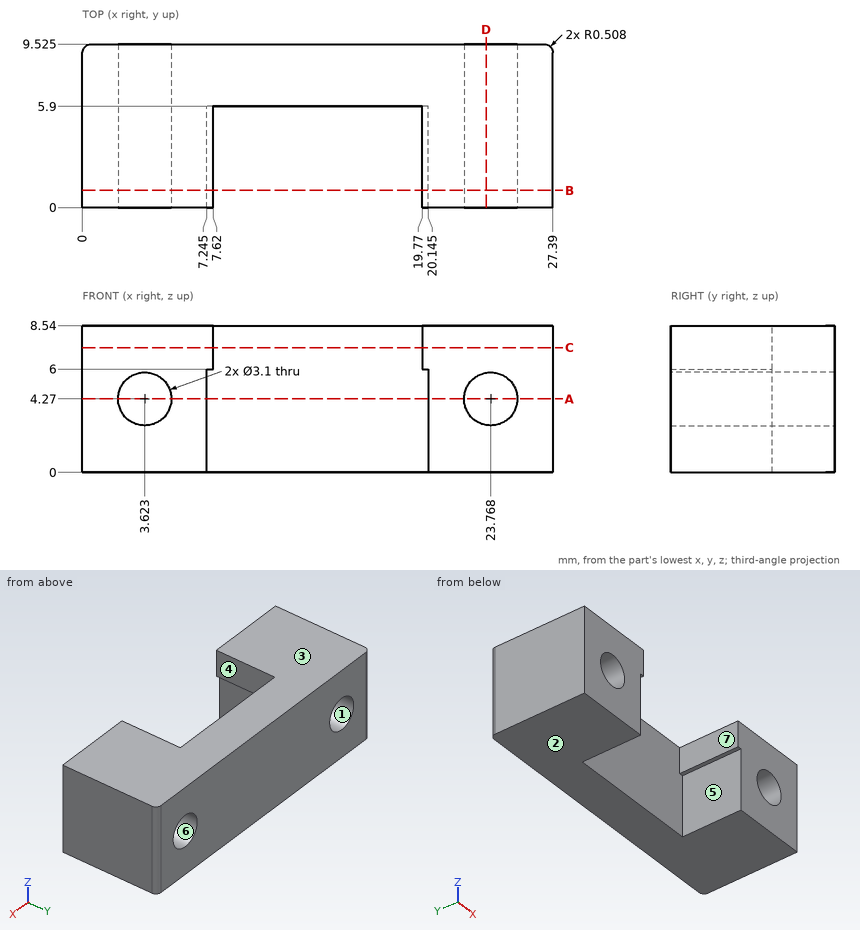
For this review, use the dimensioned drawing (mm, ordinates from the lowest corner) and the shaded views. A direction names the side the tool comes from. Coordinates: 2 decimals unless noted, no trailing zeros. Loops run counter-clockwise (first coordinate to the right, second up) from the corner with the lowest first, then second, coordinate; pieces in that order, holes last. Notation, with made-up numbers: (-31, 79.5) -> (-20, 79.5) arc R20 cw to (-20, 95.5) -> close; hole circle Ø7 at (62, 73.25). An arc over 180 degrees is marked (long way). Use a Markdown table: item, result. Add a question column.
Item 1: The part is to be moulded in two halves that separate along Z. For the marked faces 1, 2, 3 and 4, say which applies: +Z half, -Z half, draft (parallel to the pull), parting line (faces both ways), or undercut.
Item 2: Machinability: for the marked faces 5, 6 and 7, which of the approach directions +Z, -Z, +X, -X, +Y, -Y give a long, thin tool a straight path to every point of the face, cutting with its end or side? Answer none if there is none.
Item 3: We need section A-A, the plane z = 4.27. Write out the cut boundary in (x, y) (1 decimal), and give its area (3 significant figures).
Item 4: We need section C-C, the plane z = 7.25. Write out the cut boundary in (x, y) (1 decimal), and give its area (3 significant figures).
Item 5: We need section B-B, the plane y = 1. Count the separate pieces of the cut face and the enclosed holes in it.
Item 6: We need section D-D, the plane x = 23.5. Write out the cut boundary in (y, z) (1 decimal).
Item 7: Wall thickness on L1, parallel to X at y = 4.25, z = 4.27 (1 decimal); L2, parallel to X at y = 6, z = 4.27; L3, parallel to Z at x = 3.5, y = 4 (1 decimal): over which ranges is each line inside the solid? List them lowest first. Write a range as from..to.
Numbers:
| question | item | result |
|---|---|---|
| 1 | face 1 | undercut |
| 1 | face 2 | -Z half |
| 1 | face 3 | +Z half |
| 1 | face 4 | draft |
| 2 | face 5 | -Z, -Y |
| 2 | face 6 | +Y, -Y |
| 2 | face 7 | +Z, -Z, -Y |
| 3 | outline | (0, 0) -> (2.1, 0) -> (2.1, 9.5) -> (0.5, 9.5) arc R0.5 ccw to (0, 9) -> close; (5.2, 0) -> (7.2, 0) -> (7.2, 5.9) -> (20.1, 5.9) -> (20.1, 0) -> (22.2, 0) -> (22.2, 9.5) -> (5.2, 9.5) -> close; (25.3, 0) -> (27.4, 0) -> (27.4, 9) arc R0.5 ccw to (26.9, 9.5) -> (25.3, 9.5) -> close |
| 3 | area | 126 mm^2 |
| 4 | outline | (0, 0) -> (7.6, 0) -> (7.6, 5.9) -> (19.8, 5.9) -> (19.8, 0) -> (27.4, 0) -> (27.4, 9) arc R0.5 ccw to (26.9, 9.5) -> (0.5, 9.5) arc R0.5 ccw to (0, 9) -> close |
| 4 | area | 189 mm^2 |
| 5 | separate pieces | 2 |
| 5 | enclosed holes | 2 |
| 6 | outline | (0, 0) -> (9.5, 0) -> (9.5, 2.7) -> (0, 2.7) -> close; (0, 5.8) -> (9.5, 5.8) -> (9.5, 8.5) -> (0, 8.5) -> close |
| 7 | L1 | x = 0..2.1, 5.2..7.2, 20.1..22.2, 25.3..27.4 |
| 7 | L2 | x = 0..2.07, 5.17..22.22, 25.32..27.39 |
| 7 | L3 | z = 0..2.7, 5.8..8.5 |
